The model under review builds one solid part; all positions refer to its coordinate system, in mm. Face numbers are marked on the shaded views. A direction names the side the tool comes from. Coordinates: 2 decimals unless noted, no trailing zeros. Order: outer loops, then holes, each group sorted by start corner. A loop starts at its lowest first (then second) coordinate and runs counter-clockwise, first axis right, second up.
Autodesk Inventor part; units mm, degrees
ref_plane "YZ Plane" through (0, 0, 0) normal (1, 0, 0) x (0, 1, 0)
ref_plane "XZ Plane" through (0, 0, 0) normal (0, 1, 0) x (-1, 0, 0)
ref_plane "XY Plane" through (0, 0, 0) normal (0, 0, 1) x (1, 0, 0)
sketch "スケッチ1" plane through (0, 0, 0) normal (0, 0, 1) x (1, 0, 0)
  line L0 (-16, -16) -> (16, -16)
  line L1 (16, -16) -> (16, 16)
  line L2 (16, 16) -> (-16, 16)
  line L3 (-16, 16) -> (-16, -16)
  line L4 (-16, -16) -> (16, 16) construction
  line L5 (16, -16) -> (-16, 16) construction
  line L6 (-14.4, 14.4) -> (14.4, 14.4)
  line L7 (14.4, 14.4) -> (14.4, -14.4)
  line L8 (14.4, -14.4) -> (-14.4, -14.4)
  line L9 (-14.4, -14.4) -> (-14.4, 14.4)
  point P0 (0, 0)
  dimension "d0" = 32
  dimension "d1" = 32
  dimension "d2" = 1.6
extrude "押し出し1" add sketch "スケッチ1" along normal blind 180
chamfer "面取り1" distance 32 angle 45 1 edges at (-16, 0, 0)
properties part number "PipeB"
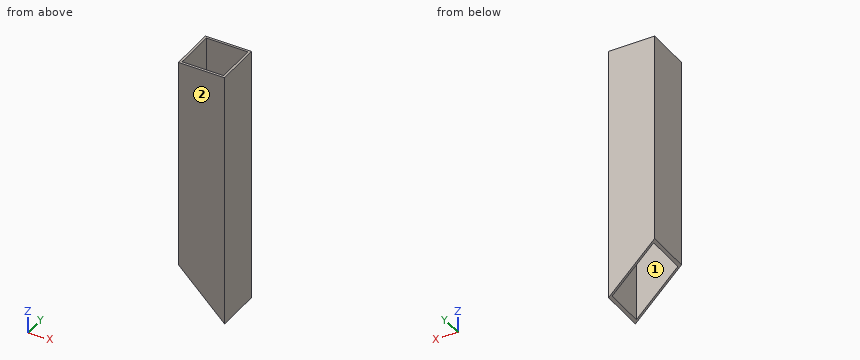
(1) For pin 1 Ø6 at (x, y) = (-8.5, 3) entering from -Z, flat-tipped, find the tip position at first contact; note if it passes through.
A:
pin 1: passes through
(2) We need section B-B, the plane z = 52. Write out the cut boundary in (x, y), and give its area (3 significant figures).
A:
outline: (-16, -16) - (16, -16) - (16, 16) - (-16, 16) - close; hole (-14.4, -14.4) - (14.4, -14.4) - (14.4, 14.4) - (-14.4, 14.4) - close
area: 195 mm2
(3) Machinability: for the marked faces 1 and 2, which of the approach directions +Z, -Z, +X, -X, +Y, -Y give a long, thin tool a straight path to every point of the face, cutting with its end or side? Answer none if there is none.
A:
face 1: +Z, -Z
face 2: +Z, -Z, +X, -X, -Y
(4) We need section A-A, the plane x = -2. Write out the cut boundary in (y, z).
A:
outline: (-16, 18) - (-14.4, 18) - (-14.4, 180) - (-16, 180) - close; (14.4, 18) - (16, 18) - (16, 180) - (14.4, 180) - close
(5) We need section C-C, the plane y = 4.5. Write out the cut boundary in (x, z).
A:
outline: (-16, 32) - (-14.4, 30.4) - (-14.4, 180) - (-16, 180) - close; (14.4, 1.6) - (16, 0) - (16, 180) - (14.4, 180) - close
(6) Wall thickness on probe 1 along X at (y, z) = (6, 55): over which ranges is the line inside the solid? List them lowest first.
A:
probe 1: x = -16 to -14.4, 14.4 to 16
